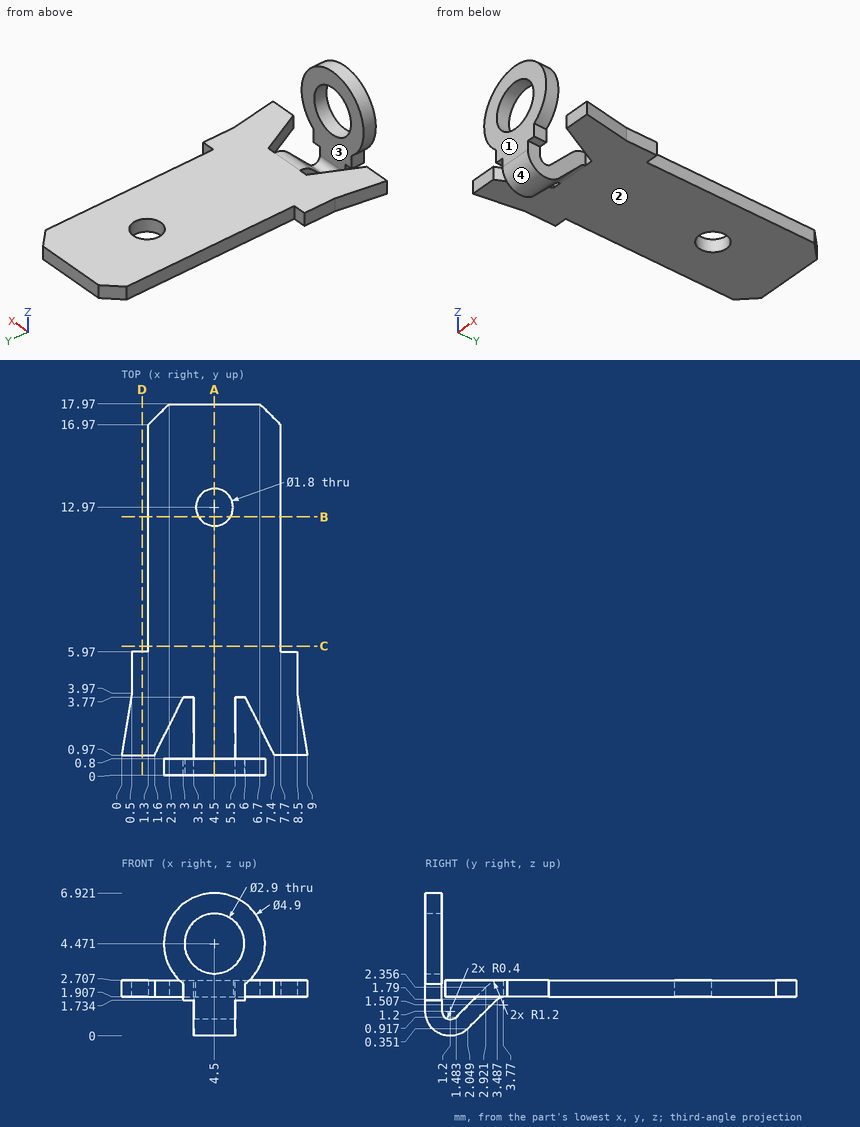
Geometry: see drawing. Coordinates: mm, zero at the bounding-box minimum. Give positions to 0.01 mm unless a question says otherwise; leave off trailing zeros. Order: outer loops, then holes, each group sorted by start corner. A loop starts at its lowest first (then second) coordinate and runs counter-clockwise, first axis right, second up.
1. Pin query (flat end, axial travel): pin 1 Ø0.9 at (x, z) = (8, 2.5) entering from -Y; pin 2 Ø3 at (x, y) = (6.5, 12.5) entering from +Z; pin 3 Ø0.6 at (y, z) = (14, 2.5) entering from +X. Return the tip coordinate at first contact, or that it passes through.
Computed:
pin 1: stops at y = 0.97
pin 2: stops at z = 2.71
pin 3: stops at x = 7.7
2. Cut plane B-B (y = 12.5). Return loops of the section in (x, z).
Computed:
outline: (1.3, 1.91) - (3.73, 1.91) - (3.73, 2.71) - (1.3, 2.71) - close; (5.27, 1.91) - (7.7, 1.91) - (7.7, 2.71) - (5.27, 2.71) - close
3. Line query: probe 1 along Y at (x, z) = (4.5, 2.4) (1 decimal); probe 2 along Z at (x, y) = (6.5, 5.5); probe 3 along Y at (x, z) = (5, 2) (1 decimal). Output: solid intervals per line, ascending.
Computed:
probe 1: y = 0 to 0.8, 3 to 12.1, 13.9 to 18
probe 2: z = 1.91 to 2.71
probe 3: y = 0 to 0.8, 2.6 to 12.2, 13.7 to 18
4. Cut plane D-D (x = 1). Return loops of the section in (y, z).
Computed:
outline: (0.97, 1.91) - (5.97, 1.91) - (5.97, 2.71) - (0.97, 2.71) - close
5. Cut plane C-C (y = 6.25). Return loops of the section in (x, z).
Computed:
outline: (1.3, 1.91) - (7.7, 1.91) - (7.7, 2.71) - (1.3, 2.71) - close
6. Cut plane A-A (x = 4.5). State how many separate pieces and enclosed holes the cut face has.
Computed:
separate pieces: 3
enclosed holes: 0
7. Draft query along Y for the marked faces 1, 2, 3 and 4. Return one class per face: released by +Y, released by -Y, zero draft, split by the parting line, or undercut.
Computed:
face 1: released by -Y
face 2: zero draft
face 3: undercut
face 4: split by the parting line
